Drawing for the job (mm, zero at the part's lowest x, y, z). A direction names the side the tool comes from. Coordinates: 2 decimals unless noted, no trailing zeros. Write each loop counter-clockwise with the first axis right and the second up, starting at its lowest first coordinate (ties: lowest second). Pieces come first, ordered by that corner, then holes. Notation, with made-up numbers: M 58,45.5 L 73,45.5 A8 cw 73,59.5 Z; hole C 59.5,11 d4. An arc over 180 degrees is marked long. Put each result on its own line as item: value. Start each with the question number.
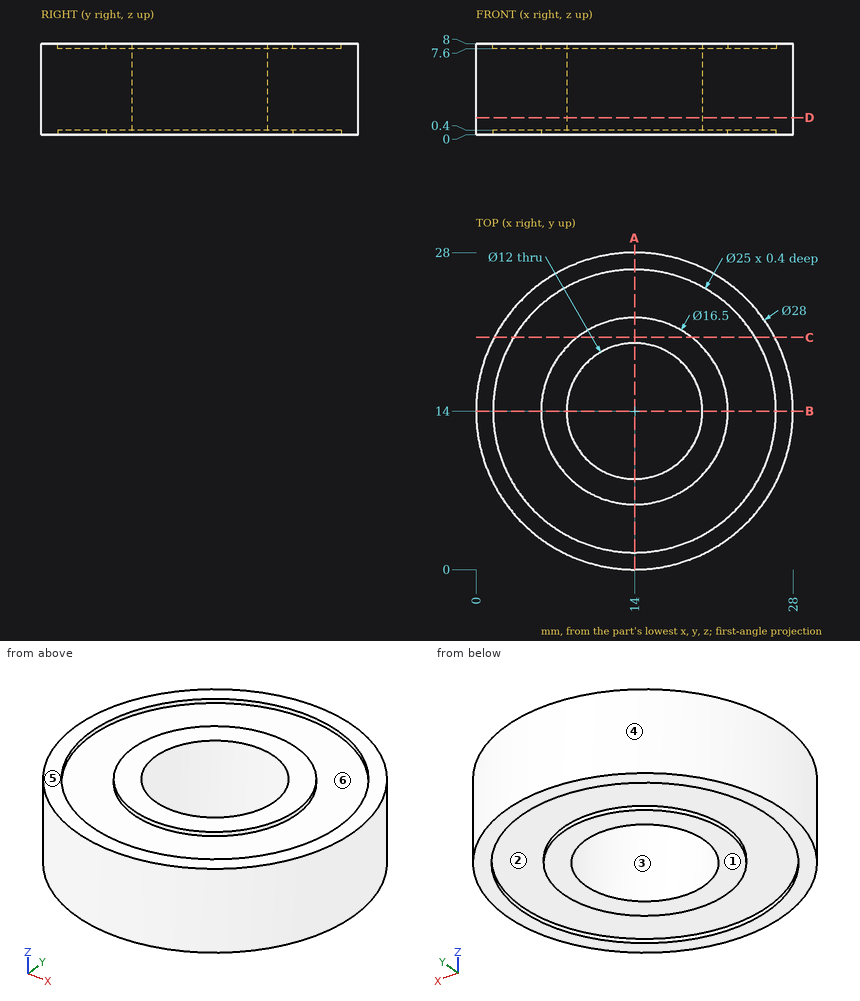
(1) Drill centre lines: line 1 (Y direction, x = 14, z = 7.85); line 2 (Y direction, x = 14, z = 2.75); line 3 (Z direction, x = 23.75, y = 18.5). Where is each one in solid material? Low to high. Write a range as [from, to].
(2) Slice it at D-D, the plane z = 1.5. Write the cut outline in (x, y), then the cut area to 3 significant figures.
(3) Two-plate mould, pull along Y, no slides. Class the marked faces 3, 4, 5 and 6: +Y half, -Y half, draft (parallel to the pull), parting line (faces both ways), or undercut.
(4) Which spindle directions (+Z, -Z, +X, -X, +Y, -Y) get a long thin tool onto all of the face, cutting with end or side? Do the marked faces 1 and 2. Say none if no direction does.
(5) Drop flat-ended pins along their axis: pin 1 (12.5 mm diameter, centred on x = 11.5, y = 11.5, fed in from +Z); pin 2 (1.5 mm diameter, centred on x = 24, y = 11, fed in from -Z); pin 3 (1 mm diameter, centred on x = 23, z = 3.5, fed in from -Y). Give the stop position or say it passes through.
(6) Slice it at A-A, the plane x = 14. Write the cut outline in (y, z), then the cut area to 3 significant figures.
(7) Slice it at C-C, the plane y = 20.5. Write the cut outline in (x, z).
Result set:
1. line 1: y = [0, 1.5], [5.75, 8], [20, 22.25], [26.5, 28]
1. line 2: y = [0, 8], [20, 28]
1. line 3: z = [0.4, 7.6]
2. outline: C 14,14 d28; hole C 14,14 d12
2. area: 503 mm^2
3. face 3: undercut
3. face 4: parting line
3. face 5: draft
3. face 6: undercut
4. face 1: -Z, +X, -X, +Y, -Y
4. face 2: -Z
5. pin 1: stops at z = 8
5. pin 2: stops at z = 0.4
5. pin 3: stops at y = 2.88
6. outline: M 0,0 L 1.5,0 L 1.5,0.4 L 5.75,0.4 L 5.75,0 L 8,0 L 8,8 L 5.75,8 L 5.75,7.6 L 1.5,7.6 L 1.5,8 L 0,8 Z; M 20,0 L 22.25,0 L 22.25,0.4 L 26.5,0.4 L 26.5,0 L 28,0 L 28,8 L 26.5,8 L 26.5,7.6 L 22.25,7.6 L 22.25,8 L 20,8 Z
6. area: 121 mm^2
7. outline: M 1.6,0 L 3.32,0 L 3.32,0.4 L 8.92,0.4 L 8.92,0 L 19.08,0 L 19.08,0.4 L 24.68,0.4 L 24.68,0 L 26.4,0 L 26.4,8 L 24.68,8 L 24.68,7.6 L 19.08,7.6 L 19.08,8 L 8.92,8 L 8.92,7.6 L 3.32,7.6 L 3.32,8 L 1.6,8 Z
